Work out the finished part from the listing and answer in its coordinate system (mm). Face numbers are marked on the shaded views. Round coordinates to 2 decimals unless told otherwise and drop trailing zeros. Write each loop counter-clockwise with the first axis right and the second up, starting at its lowest first coordinate (ties: lowest second). Pieces come first, ordered by that corner, then holes.
1. Straight lines are drawn through the part: probe 1 along Y at (x, z) = (21.5, 11.75); probe 2 along Z at (x, y) = (7.5, -9); probe 3 along X at (y, z) = (-23, 9.75) (3 decimals). For each, find the intervals that lie inside material, in ascending order.
2. Flat-ended cylindrical pins translate along their axes: pin 1 Ø7 at (x, y) = (11.5, -12.5) entering from +Z; pin 2 Ø8 at (y, z) = (-2.5, 6) entering from +X; pin 3 Ø5 at (y, z) = (-17, 12.5) entering from +X. Find the tip coordinate at first contact, or state that the pin passes through.
3. Find section C-C (y = -13). Write down the section's boundary in (x, z).
4. Determine the mould class of the marked faces 1, 2, 3 and 4 for opening direction X: pulls with the +X half, pulls with the -X half, needs draft (parallel to the pull), parting line crosses it, or undercut.
5. Find section D-D (z = 9.5). Write down the section's boundary in (x, y), and give its area (3 significant figures).
6. Find section A-A (z = 17). Write down the section's boundary in (x, y), and give its area (3 significant figures).
7. Find section B-B (x = 21). Write down the section's boundary in (y, z), and give its area (3 significant figures).
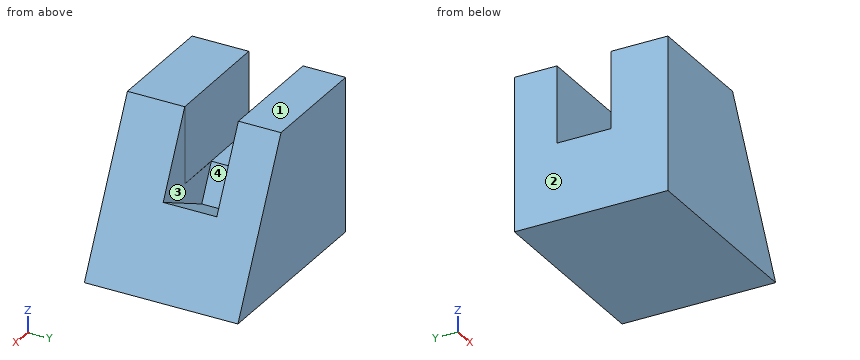
```python
from build123d import *

# Parameters (mm, degrees)
F1_DEPTH = 25.4
F2_W     = 8.867607
F2_H     = 14.199032
F3_DEPTH = 12.7
F5_DEPTH = 12.7


with BuildPart() as f1:
    # F0 (on Front) → F1 (new body)
    with BuildSketch(Plane.XZ):
        Polygon((0, 25.4), (0, 0), (31.75, 0), (19.05, 25.4), align=None)
    extrude(amount=F1_DEPTH)

    # F2 (on face) → F3 (cut, symmetric)
    with BuildSketch(Plane(origin=(25.4, 0, 12.7), x_dir=(0, 1, 0), z_dir=(0.894427, 0, 0.447214))):
        with Locations((-11.487583, 7.099516)):
            Rectangle(F2_W, F2_H)
    extrude(amount=F3_DEPTH, both=True, mode=Mode.SUBTRACT)

    # F4 (on face) → F5 (cut, symmetric)
    with BuildSketch(Plane.XY.offset(25.4)):
        Polygon((19.05, -15.921386), (19.05, -7.053779), (0, -7.053779), (0, -16.022153), align=None)
    extrude(amount=F5_DEPTH, both=True, mode=Mode.SUBTRACT)


solid = f1.part
```
Worked answers:
1. probe 1: y = -25.4 to -15.92, -7.05 to 0
1. probe 2: z = 0 to 12.7
1. probe 3: x = 0 to 26.875
2. pin 1: stops at z = 25.4
2. pin 2: stops at x = 30.75
2. pin 3: stops at x = 26.75
3. outline: (0, 0) - (31.75, 0) - (25.4, 12.7) - (14.04, 7.02) - (11.2, 12.7) - (0, 12.7) - close
4. face 1: needs draft
4. face 2: pulls with the -X half
4. face 3: undercut
4. face 4: undercut
5. outline: (0, -25.4) - (27, -25.4) - (27, 0) - (0, 0) - close; hole (12.8, -15.92) - (19, -15.92) - (19, -7.05) - (12.8, -7.05) - close
5. area: 631 mm2
6. outline: (0, -25.4) - (23.25, -25.4) - (23.25, -15.92) - (19.05, -15.92) - (0, -16.02) - close; (0, -7.05) - (23.25, -7.05) - (23.25, 0) - (0, 0) - close
6. area: 383 mm2
7. outline: (-25.4, 0) - (0, 0) - (0, 21.5) - (-7.05, 21.5) - (-7.05, 10.5) - (-15.92, 10.5) - (-15.92, 21.5) - (-25.4, 21.5) - close
7. area: 449 mm2
